Input: part model. Units: mm. Frame: model coordinates. Round coordinates to 2 decimals unless told otherwise and drop trailing zeros. One line per question, with ' | ' between items. Start each with the question number.
Item 1: Section A-A, the plane y = 0.3. Give the number of separate pieces and of enclosed holes in the cut face, plus the area to 3 significant figures.
Item 2: First-contact query: pin 1 (2 mm diameter, centred on x = -90, z = -25, fed in from -Y). Flat tip, straight axial feed; report the tip coordinate or a pass-through.
Item 3: Material intervals for line 1 along X through (y, z) = (0.35, -8); line 2 along X through (y, z) = (0.4, -25); line 3 along Z through (x, y) = (-90, 1.05), sorted ascending.
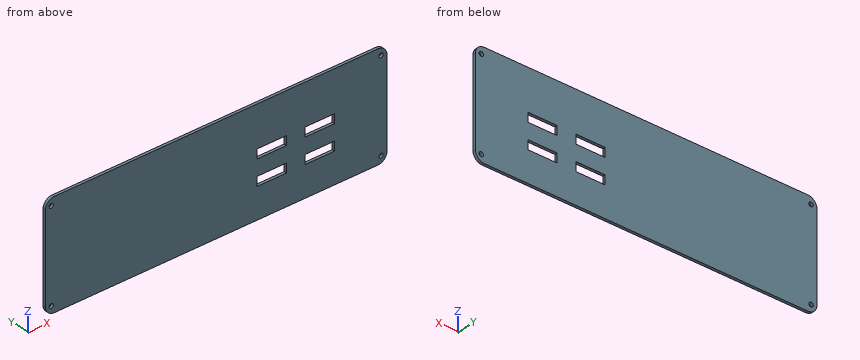
```python
from build123d import *

# Parameters (mm, degrees)
SKETCH1_W                      = 186.5
SKETCH1_H                      = 58
BOSS_EXTRUDE1_DEPTH            = 1.5
FILLET1_R                      = 5
M2_CLEARANCE_HOLE1_D           = 2.4
M2_CLEARANCE_HOLE1_CSINK_D     = 2.45
M2_CLEARANCE_HOLE1_CSINK_ANGLE = 90
SKETCH4_W                      = 16
SKETCH4_H                      = 5.015455786
CUT_EXTRUDE1_DEPTH             = 98.666844425


with BuildPart() as part:
    # Sketch1 → Boss-Extrude1 (new body)
    with BuildSketch(Plane(origin=(0, 0, 0), x_dir=(1, 0, 0), z_dir=(0, 1, 0))):
        Rectangle(SKETCH1_W, SKETCH1_H)
    extrude(amount=BOSS_EXTRUDE1_DEPTH)

    # Fillet1
    fillet1_edges = [part.edges().sort_by_distance(p)[0] for p in [
        (-93.25, 0.75, -29),
        (93.25, 0.75, -29),
        (93.25, 0.75, 29),
        (-93.25, 0.75, 29),
    ]]
    fillet(fillet1_edges, radius=FILLET1_R)

    # M2 Clearance Hole1 (through all)
    with Locations(Plane(origin=(0, 1.5, 0), x_dir=(1, 0, 0), z_dir=(0, 1, 0))):
        with Locations((-90, 25), (90, 25), (90, -25), (-90, -25)):
            CounterSinkHole(M2_CLEARANCE_HOLE1_D / 2, M2_CLEARANCE_HOLE1_CSINK_D / 2, counter_sink_angle=M2_CLEARANCE_HOLE1_CSINK_ANGLE)

    # Sketch4 → Cut-Extrude1 (cut, through all)
    with BuildSketch(Plane(origin=(0, 1.5, 0), x_dir=(1, 0, 0), z_dir=(0, 1, 0))):
        with Locations((30.376648893, 9.645107281)):
            Rectangle(SKETCH4_W, SKETCH4_H)
        with Locations((56.611340698, 9.645107281)):
            Rectangle(SKETCH4_W, SKETCH4_H)
        with Locations((30.376648893, -4.050945058)):
            Rectangle(SKETCH4_W, SKETCH4_H)
        with Locations((56.611340698, -4.050945058)):
            Rectangle(SKETCH4_W, SKETCH4_H)
    extrude(amount=-CUT_EXTRUDE1_DEPTH, mode=Mode.SUBTRACT)


solid = part.part
```
Return value:
1) separate pieces: 1 | enclosed holes: 8 | area: 10,500 mm2
2) pin 1: through
3) line 1: -93.25 to 22.38, 38.38 to 48.61, 64.61 to 93.25 | line 2: -93.15 to -91.2, -88.8 to 88.8, 91.2 to 93.15 | line 3: -28.68 to -26.2, -23.8 to 23.8, 26.2 to 28.68
